```python
from build123d import *

# Parameters (mm, degrees)
SKETCH1_W           = 30
SKETCH1_H           = 20
BOSS_EXTRUDE1_DEPTH = 20


with BuildPart() as part:
    # Sketch1 → Boss-Extrude1 (new body)
    with BuildSketch(Plane.XY):
        Polygon((-40, -25), (40, -25), (55, -25), (55, -15), (40, -15), (40, 15), (55, 15), (55, 25), (40, 25), (-40, 25), (-55, 25), (-55, 15), (-40, 15), (-40, -15), (-55, -15), (-55, -25), align=None)
        Rectangle(SKETCH1_W, SKETCH1_H, mode=Mode.SUBTRACT)
    extrude(amount=BOSS_EXTRUDE1_DEPTH)


solid = part.part
```
Check sheet for the modelled part. Datum: model origin and axes. Units: mm. A direction names the side the tool comes from. Give positions to 0.01 mm unless a question says otherwise; leave off trailing zeros. Write each loop counter-clockwise with the first axis right and the second up, starting at its lowest first coordinate (ties: lowest second). Pieces come first, ordered by that corner, then holes. Notation, with made-up numbers: (67.25, 64) - (106.25, 64) arc R24 cw to (106.25, 97) - close; hole circle Ø2 at (54, 8). An arc over 180 degrees is marked (long way). Answer as a JSON object with one key per item and string values. Group by question number.
1) Sectioned sample at B-B (z = 4). Record the cut outline in (x, y).
2) Access from +Z, -Z, +X, -X, +Y, -Y to the whole of each face (thin tool, end or side, straight path). Record for faces 1 (the face through (-1, 11, 0)), 2 (the face through (-55, 20, 10)), 3 (the face through (-47, -15, 10)), 4 (the face through (47, 15, 10)), 5 (the face through (-15, 0, 10)).
3) Sectioned sample at C-C (x = -47). Record the cut outline in (y, z).
4) Sectioned sample at D-D (y = -14). Record the cut outline in (x, z), then the cut area to 3 significant figures.
5) Sectioned sample at A-A (x = -6). Record the cut outline in (y, z).
6) Release check for a two-part mould opening along X. For faces 6 (the face through (15, 0, 10)), 7 (the face through (-55, -20, 10)), 8 (the face through (0, 10, 10)), 9 (the face through (-48, 15, 10)) record: pulls with the +X half, pulls with the -X half, needs draft (parallel to the pull), parting line crosses it, or undercut.
7) Depth check by flat-ended pin: P1, Ø10, axis at y = -2, z = 8, coming from the +X side; P2, Ø6, axis at x = 43.5, y = 2.5, coming from the +Z side; P3, Ø6, axis at y = 11.5, z = 7.5, coming from the -X side. Enter the tip coordinate at first touch or a pass-through.
8) Thickness scan on probe 1 along X at (y, z) = (-3, 11.75); probe 2 along Y at (x, z) = (-5.5, 2.5); probe 3 along Y at (x, z) = (-49.5, 12.25). Record the ranges inside material, lowest first. Write a range as from..to.
Geometry results:
{
 "1": {"outline": "(-55, -25) - (55, -25) - (55, -15) - (40, -15) - (40, 15) - (55, 15) - (55, 25) - (-55, 25) - (-55, 15) - (-40, 15) - (-40, -15) - (-55, -15) - close; hole (-15, -10) - (15, -10) - (15, 10) - (-15, 10) - close"},
 "2": {"face 1": "-Z, +X, -X, +Y, -Y", "face 2": "+Z, -Z, -X, +Y, -Y", "face 3": "+Z, -Z, -X", "face 4": "+Z, -Z, +X", "face 5": "+Z, -Z"},
 "3": {"outline": "(-25, 0) - (-15, 0) - (-15, 20) - (-25, 20) - close; (15, 0) - (25, 0) - (25, 20) - (15, 20) - close"},
 "4": {"outline": "(-40, 0) - (40, 0) - (40, 20) - (-40, 20) - close", "area": "1,600 mm^2"},
 "5": {"outline": "(-25, 0) - (-10, 0) - (-10, 20) - (-25, 20) - close; (10, 0) - (25, 0) - (25, 20) - (10, 20) - close"},
 "6": {"face 6": "undercut", "face 7": "pulls with the -X half", "face 8": "undercut", "face 9": "needs draft"},
 "7": {"P1": "stops at x = 40", "P2": "passes through", "P3": "stops at x = -40"},
 "8": {"probe 1": "x = -40..-15, 15..40", "probe 2": "y = -25..-10, 10..25", "probe 3": "y = -25..-15, 15..25"}
}
